```python
from build123d import *

# Parameters (mm, degrees)
F0_R      = 8.25
F1_DEPTH  = 5
F2_T      = -0.8
F3_R      = 3.75
F4_DEPTH  = 25
F5_R      = 8.25
F6_DEPTH  = 5
F7_SIZE   = 5
F8_T      = 2.3
F9_R      = 2.5
F10_DEPTH = 25


# Not quite as in the source:
# - a shell that OpenCascade refuses in one call is made with other operations: the cavity is built on its own and cut out


with BuildPart() as f1:
    # F0 (on Top) → F1 (new body)
    with BuildSketch(Plane.XY):
        Circle(F0_R)
    extrude(amount=F1_DEPTH)

    # F2
    f2_openings = [f1.faces().sort_by_distance(p)[0] for p in [
        (0, 0, 5),
    ]]
    offset(amount=F2_T, openings=f2_openings)

    # F3 (on face) → F4 (cut)
    with BuildSketch(Plane.XY.offset(0.8)):
        Circle(F3_R)
    extrude(amount=-F4_DEPTH, mode=Mode.SUBTRACT)

    # F5 (on face) → F6 (join)
    with BuildSketch(Plane.XY.offset(5)):
        Circle(F5_R)
    extrude(amount=F6_DEPTH)

    # F7
    f7_edges = [f1.edges().sort_by_distance(p)[0] for p in [
        (-8.25, 0, 10),
    ]]
    chamfer(f7_edges, length=F7_SIZE)

    # F8: shell of thickness 2.3, made by hand


with BuildPart() as f8_core1:
    # F8_t2: copy of F1
    add(f1.part)

    # the walls: a layer under each face that stays
    f8_faces = [f8_core1.faces().sort_by_distance(p)[0] for p in [
        (-8.25, 0, 2.5),
        (-5.75, 0, 7.5),
        (-5.5, -5.5, 0),
        (0, 0, 10),
        (-3.75, 0, 0.4),
        (-4.9666666667, -4.9666666667, 0.8),
        (-7.45, 0, 2.9),
    ]]
    thicken(f8_faces, amount=-F8_T, mode=Mode.SUBTRACT)

    # F8_s3 → F8_t4 (revolve, cut)
    with BuildSketch(Plane.XZ):
        Polygon((7.427, 0.823), (7.45, -1.5), (9.75, -1.5), (9.75, 0.8), align=None)
    revolve(axis=Axis((0, 0, 0.8), (0, 0, -1)), mode=Mode.SUBTRACT)


with BuildPart() as f1_1:
    add(f1.part)

    # what is left inside the walls is the cavity
    f8_cavity = [f8_core1.part.solids().sort_by_distance(p)[0] for p in [
        (-4.081045, 0, 5.883737),
    ]]
    add(f8_cavity, mode=Mode.SUBTRACT)

    # F9 (on face) → F10 (cut)
    with BuildSketch(Plane.XY.offset(10)):
        Circle(F9_R)
    extrude(amount=-F10_DEPTH, mode=Mode.SUBTRACT)


solid = f1_1.part
```
Work out the finished part from the listing and answer in its coordinate system (mm). A direction names the side the tool comes from. Give positions to 0.01 mm unless a question says otherwise; leave off trailing zeros. Loops run counter-clockwise (first coordinate to the right, second up) from the corner with the lowest first, then second, coordinate; pieces in that order, holes last. Notation, with made-up numbers: (75.5, -33.75) -> (116.5, -33.75) arc R8 ccw to (116.5, -29.75) -> close; hole circle Ø3 at (-17, 4). An arc over 180 degrees is marked (long way). One line per question, with ' | ' between items. Start each with the question number.
1) Section C-C, the plane z = 4 is taken. Determine the outline of the cut face in (x, y).
2) Determine the mould class of faces 4 (the face through (2, -5, 5)), 5 (the face through (2, -2, 10)), 6 (the face through (7.62, -3.16, 2.46)) for opening direction Y: +Y half, -Y half, draft (parallel to the pull), parting line (faces both ways), or undercut.
3) Section A-A, the plane x = 0 is taken. Determine the outline of the cut face in (y, z), then the cut area to 3 significant figures.
4) Straight lines are drawn through the part: L1, parallel to Y at x = 0, z = 2.05; L2, parallel to Y at x = 0, z = 8.25; L3, parallel to Z at x = 4.25, y = -4. For each, find the intervals that lie inside material, in ascending order.
5) Section D-D, the plane z = 7 is taken. Determine the outline of the cut face in (x, y), then the cut area to 3 significant figures.
6) Each of these flat-tipped pins is pushed along its axis until it touches: pin 1 (3 mm diameter, centred on x = 3, y = -6, fed in from +Z); pin 2 (2 mm diameter, centred on x = 1.5, z = 2, fed in from +Y); pin 3 (1 mm diameter, centred on y = 6, z = 4.5, fed in from -X); pin 4 (4.5 mm diameter, centred on x = 0, y = 0, fed in from -Z). Where does it stop, or does it pass through?
7) For faces 1 (the face through (2, -4, 0)), 2 (the face through (3, -3, 0.8)), 3 (the face through (-3.746, 0.165, 0.406)), determine the directions among +Z, -Z, +X, -X, +Y, -Y from which every point of the face is accessible in a straight line to the end or side of a thin tool.
Resolved:
1) outline: circle Ø16.5 at (0, 0); hole circle Ø14.9 at (0, 0)
2) face 4: undercut | face 5: draft | face 6: parting line
3) outline: (-8.25, 0) -> (-3.75, 0) -> (-3.75, 0.8) -> (-7.45, 0.8) -> (-7.45, 5) -> (-5, 5) -> (-2.5, 7.5) -> (-2.5, 10) -> (-3.25, 10) -> (-8.25, 5) -> close; (2.5, 7.5) -> (5, 5) -> (7.45, 5) -> (7.45, 0.8) -> (3.75, 0.8) -> (3.75, 0) -> (8.25, 0) -> (8.25, 5) -> (3.25, 10) -> (2.5, 10) -> close | area: 40.2 mm2
4) L1: -8.25 to -7.45, 7.45 to 8.25 | L2: -5 to -2.5, 2.5 to 5 | L3: 0 to 0.8, 5 to 7.41
5) outline: circle Ø12.5 at (0, 0); hole circle Ø5.99 at (0, 0) | area: 94.5 mm2
6) pin 1: z = 8.04 | pin 2: y = 8.23 | pin 3: x = -6.15 | pin 4: through
7) face 1: -Z, +X, -X, +Y, -Y | face 2: none | face 3: -Z
